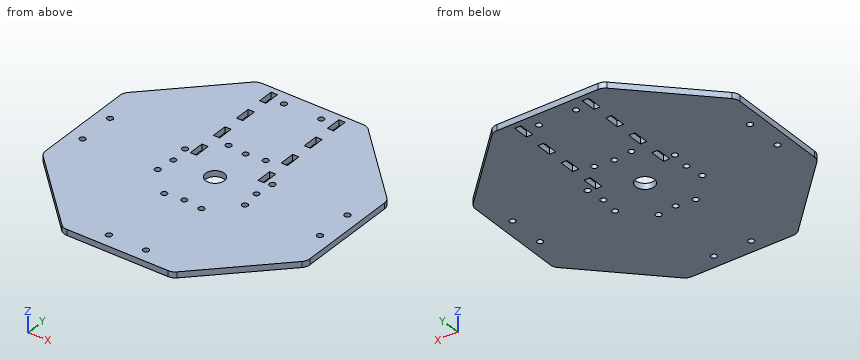
```python
from build123d import *

# Parameters (mm, degrees)
F0_R     = 1.5
F0_R_2   = 1.45
F0_W     = 3.18
F0_H     = 8
F0_R_3   = 4.75
F1_DEPTH = 3
F2_R     = 5


with BuildPart() as f1:
    # F0 (on Top) → F1 (new body)
    with BuildSketch(Plane.XY):
        Polygon((67.5, 27.96), (27.96, 67.5), (-27.96, 67.5), (-67.5, 27.96), (-67.5, -27.96), (-27.96, -67.5), (27.96, -67.5), (67.5, -27.96), align=None)
        with Locations((-9.5, -60.598515)):
            Circle(F0_R, mode=Mode.SUBTRACT)
        with Locations((-60.598515, -9.5)):
            Circle(F0_R, mode=Mode.SUBTRACT)
        with Locations((-9.5, -22.265932)):
            Circle(F0_R, mode=Mode.SUBTRACT)
        with Locations((-22.265932, -9.5)):
            Circle(F0_R, mode=Mode.SUBTRACT)
        with Locations((9.5, -60.598515)):
            Circle(F0_R, mode=Mode.SUBTRACT)
        with Locations((0, -21.215)):
            Circle(F0_R_2, mode=Mode.SUBTRACT)
        with Locations((9.5, -22.265932)):
            Circle(F0_R, mode=Mode.SUBTRACT)
        with Locations((22.265932, -9.5)):
            Circle(F0_R, mode=Mode.SUBTRACT)
        with Locations((60.598515, -9.5)):
            Circle(F0_R, mode=Mode.SUBTRACT)
        with Locations((-60.598515, 9.5)):
            Circle(F0_R, mode=Mode.SUBTRACT)
        with Locations((-21.215, 0)):
            Circle(F0_R_2, mode=Mode.SUBTRACT)
        with Locations((-22.265932, 9.5)):
            Circle(F0_R, mode=Mode.SUBTRACT)
        with Locations((-17.29, 12.5)):
            Rectangle(F0_W, F0_H, mode=Mode.SUBTRACT)
        with Locations((-17.29, 28.5)):
            Rectangle(F0_W, F0_H, mode=Mode.SUBTRACT)
        with Locations((-9.5, 22.265932)):
            Circle(F0_R, mode=Mode.SUBTRACT)
        with Locations((-17.29, 44.5)):
            Rectangle(F0_W, F0_H, mode=Mode.SUBTRACT)
        with Locations((-17.29, 60.5)):
            Rectangle(F0_W, F0_H, mode=Mode.SUBTRACT)
        with Locations((-9.5, 60.598515)):
            Circle(F0_R, mode=Mode.SUBTRACT)
        Circle(F0_R_3, mode=Mode.SUBTRACT)
        with Locations((21.215, 0)):
            Circle(F0_R_2, mode=Mode.SUBTRACT)
        with Locations((17.29, 12.5)):
            Rectangle(F0_W, F0_H, mode=Mode.SUBTRACT)
        with Locations((22.265932, 9.5)):
            Circle(F0_R, mode=Mode.SUBTRACT)
        with Locations((0, 21.215)):
            Circle(F0_R_2, mode=Mode.SUBTRACT)
        with Locations((9.5, 22.265932)):
            Circle(F0_R, mode=Mode.SUBTRACT)
        with Locations((17.29, 28.5)):
            Rectangle(F0_W, F0_H, mode=Mode.SUBTRACT)
        with Locations((60.598515, 9.5)):
            Circle(F0_R, mode=Mode.SUBTRACT)
        with Locations((17.29, 44.5)):
            Rectangle(F0_W, F0_H, mode=Mode.SUBTRACT)
        with Locations((9.5, 60.598515)):
            Circle(F0_R, mode=Mode.SUBTRACT)
        with Locations((17.29, 60.5)):
            Rectangle(F0_W, F0_H, mode=Mode.SUBTRACT)
    extrude(amount=F1_DEPTH)

    # F2
    f2_edges = [f1.edges().sort_by_distance(p)[0] for p in [
        (-27.96, 67.5, 1.5),
        (-67.5, 27.96, 1.5),
        (-67.5, -27.96, 1.5),
        (-27.96, -67.5, 1.5),
        (27.96, -67.5, 1.5),
        (67.5, -27.96, 1.5),
        (67.5, 27.96, 1.5),
        (27.96, 67.5, 1.5),
    ]]
    fillet(f2_edges, radius=F2_R)


solid = f1.part
```
The model under review builds one solid part; all positions refer to its coordinate system, in mm. Round coordinates to 2 decimals unless told otherwise and drop trailing zeros. Order: outer loops, then holes, each group sorted by start corner. A loop starts at its lowest first (then second) coordinate and runs counter-clockwise, first axis right, second up. Notation, with made-up numbers: (-36.5, 76) -> (-5.5, 76) arc R32 cw to (-5.5, 110) -> close; hole circle Ø4 at (-32, 30.5). An arc over 180 degrees is marked (long way). Use a Markdown table: item, result.
Q1. We need section B-B on z = 0.85. State how many separate pieces and enclosed holes the cut face has, then the cut area to 3 significant figures.
Values:
| item | result |
|---|---|
| separate pieces | 1 |
| enclosed holes | 29 |
| area | 14,700 mm^2 |
Q2. Clearance check with flat-ended pins moving along their axes: P1, Ø1.5, axis at y = 45, z = 2, coming from the -X side; P2, Ø1, axis at x = 27.5, z = 1.5, coming from the +Y side (3 decimals); P3, Ø2.5, axis at x = 9.5, y = 60.6, coming from the -Z side. State where each tip first meets the part, or that it passes through.
Values:
| item | result |
|---|---|
| P1 | stops at x = -51.21 |
| P2 | stops at y = 67.375 |
| P3 | passes through |
Q3. We need section A-A on y = -44. Write out the cut boundary in (x, z).
Values:
| item | result |
|---|---|
| outline | (-51.46, 0) -> (51.46, 0) -> (51.46, 3) -> (-51.46, 3) -> close |
Q4. For line 1 (X direction, y = 16, z = 0.2); line 2 (Y direction, x = 18, z = 2.3); line 3 (Y direction, x = -9.5, z = 1.8), list the stretches that pass through material, from the lowest coordinate up.
Values:
| item | result |
|---|---|
| line 1 | x = -67.5 to -18.88, -15.7 to 15.7, 18.88 to 67.5 |
| line 2 | y = -67.5 to 8.5, 16.5 to 24.5, 32.5 to 40.5, 48.5 to 56.5, 64.5 to 67.5 |
| line 3 | y = -67.5 to -62.1, -59.1 to -23.77, -20.77 to 20.77, 23.77 to 59.1, 62.1 to 67.5 |
Q5. We need section C-C on x = -46. Write out the cut boundary in (y, z).
Values:
| item | result |
|---|---|
| outline | (-49.46, 0) -> (49.46, 0) -> (49.46, 3) -> (-49.46, 3) -> close |
